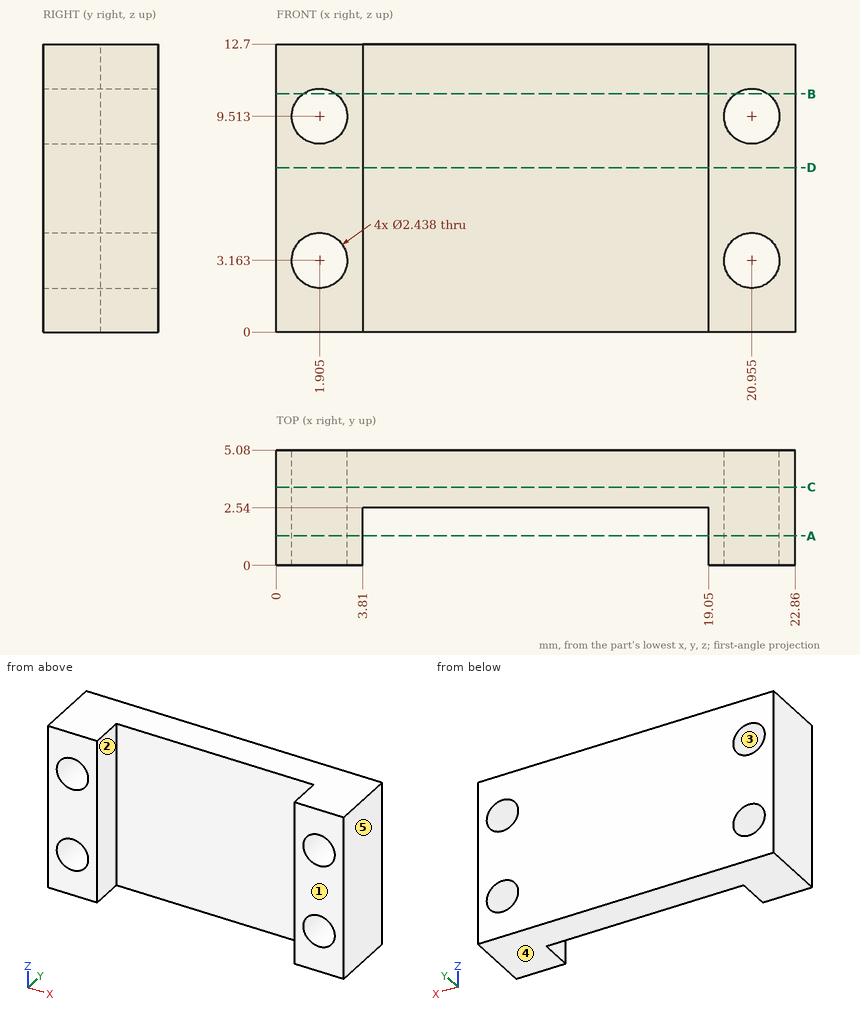
Drawing for the job (mm, zero at the part's lowest x, y, z). A direction names the side the tool comes from. Coordinates: 2 decimals unless noted, no trailing zeros. Write each loop counter-clockwise with the first axis right and the second up, starting at its lowest first coordinate (ties: lowest second). Pieces come first, ordered by that corner, then holes. Notation, with made-up numbers: (-20.75, 57) -> (3.25, 57) arc R23 ccw to (3.25, 74) -> close; hole circle Ø1 at (72, 83). An arc over 180 degrees is marked (long way). One line per item, written item: value. Start each with the question number.
1) Which spindle directions (+Z, -Z, +X, -X, +Y, -Y) get a long thin tool onto all of the face, cutting with end or side? Do the marked faces 1 and 2. Say none if no direction does.
2) Slice it at A-A on y = 1.3. Count the separate pieces of the cut face and the enclosed holes in it.
3) Slice it at D-D on z = 7.25. Write the cut outline in (x, y).
4) Slice it at B-B on z = 10.5. Write the cut outline in (x, y).
5) Probe probe 1 along X at (y, z) = (2.45, 9); probe 2 along Z at (x, y) = (1.5, 4.15); probe 3 along X at (y, z) = (4, 9). List the from-to ranges inside material, lowest first.
6) Pull direction Z, two halves, no side cores. Call the marked faces 3, 4 and 5: +Z half, -Z half, draft (parallel to the pull), parting line (faces both ways), or undercut.
7) Flat gauge pin, fed straight in: pin 1 Ø2 at (x, z) = (1.9, 3.16) entering from +Y. Where does the tip first touch, or does it go through?
8) Slice it at C-C on y = 3.45. Write the cut outline in (x, z) (1 decimal), then the cut area to 3 significant figures.
Answers follow:
1. face 1: +Z, -Z, +X, -X, -Y
1. face 2: +Z, -Z, -Y
2. separate pieces: 2
2. enclosed holes: 4
3. outline: (0, 0) -> (3.81, 0) -> (3.81, 2.54) -> (19.05, 2.54) -> (19.05, 0) -> (22.86, 0) -> (22.86, 5.08) -> (0, 5.08) -> close
4. outline: (0, 0) -> (1.19, 0) -> (1.19, 5.08) -> (0, 5.08) -> close; (2.62, 0) -> (3.81, 0) -> (3.81, 2.54) -> (19.05, 2.54) -> (19.05, 0) -> (20.24, 0) -> (20.24, 5.08) -> (2.62, 5.08) -> close; (21.67, 0) -> (22.86, 0) -> (22.86, 5.08) -> (21.67, 5.08) -> close
5. probe 1: 0 to 0.8, 3.01 to 3.81, 19.05 to 19.85, 22.06 to 22.86
5. probe 2: 0 to 2.01, 4.31 to 8.36, 10.66 to 12.7
5. probe 3: 0 to 0.8, 3.01 to 19.85, 22.06 to 22.86
6. face 3: undercut
6. face 4: -Z half
6. face 5: draft
7. pin 1: through
8. outline: (0, 0) -> (22.9, 0) -> (22.9, 12.7) -> (0, 12.7) -> close; hole circle Ø2.4 at (1.9, 3.2); hole circle Ø2.4 at (1.9, 9.5); hole circle Ø2.4 at (21, 3.2); hole circle Ø2.4 at (21, 9.5)
8. area: 272 mm2
